Could you check a few things on this model? Use its own coordinates, in mm. Face numbers are marked on the shaded views. A direction names the side the tool comes from. Give positions to 0.01 mm unless a question says otherwise; leave off trailing zeros. Answer in a Markdown table with one row per item. Add a question column.
1. I need wall thicknesses on line 1 along Z through (x, y) = (-3.25, 29.5); line 2 along X through (y, z) = (18.5, -8.25); line 3 along X through (y, z) = (22, -2.5). Which ranges of each line are inside material? Lowest first, please. Write a range as from..to.
2. Thinking about a two-plate mould opening in Z: for the marked faces 3, 4, 5 and 6, which applies, released by +Z, released by -Z, zero draft, split by the parting line, or undercut?
3. Which directions (+Z, -Z, +X, -X, +Y, -Y) give clear straight access to the entire face, cutting with the end or side of a thin tool? Please do the marked faces 1 and 2.
4. I'm going to push flat-ended pins straight in: pin 1 Ø3.5 at (y, z) = (44.5, -1) entering from -X; pin 2 Ø0.5 at (y, z) = (30.5, -9) entering from +X; pin 3 Ø3.5 at (x, y) = (0, 21) entering from +Z. Where does each tip first touch, or does it pass through?
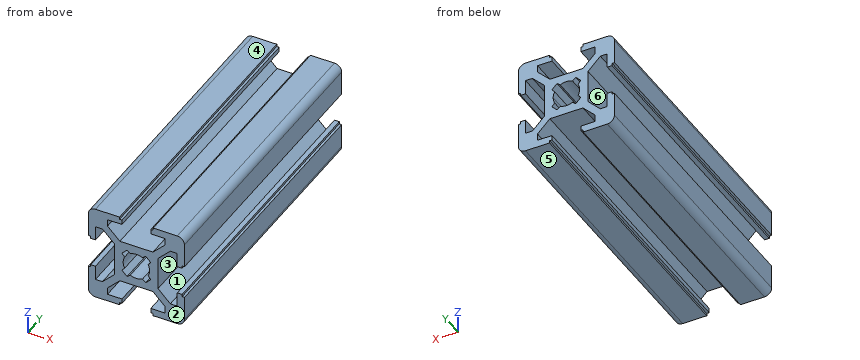
```python
from build123d import *

# Parameters (mm, degrees)
DODANIE_WYCI_GNI_CIE1_DEPTH = 60


with BuildPart() as part:
    # Szkic1 → Dodanie-wyciągnięcie1 (new body)
    with BuildSketch(Plane(origin=(0, 0, 0), x_dir=(1, 0, 0), z_dir=(0, 1, 0))):
        with BuildLine():
            Line((-7.06, 6), (-4.5, 3.440546933))
            Line((-4.5, 3.440546933), (-4.5, 4.5))
            Line((-4.5, 4.5), (-3.440546933, 4.5))
            Line((-3.440546933, 4.5), (-6, 7.06))
            Line((-6, 7.06), (-6, 8.5))
            Line((-6, 8.5), (-3, 8.5))
            Line((-3, 8.5), (-3, 9.5))
            Line((-3, 9.5), (-3.5, 9.5))
            Line((-3.5, 9.5), (-3.5, 10))
            Line((-3.5, 10), (-8.5, 10))
            ThreePointArc((-8.5, 10), (-9.560660172, 9.560660172), (-10, 8.5))
            Line((-10, 8.5), (-10, 3.5))
            Line((-10, 3.5), (-9.5, 3.5))
            Line((-9.5, 3.5), (-9.5, 3))
            Line((-9.5, 3), (-8.5, 3))
            Line((-8.5, 3), (-8.5, 6))
            Line((-8.5, 6), (-7.06, 6))
        make_face()
        with BuildLine():
            Line((4.5, 4.5), (4.5, 3.440546933))
            Line((4.5, 3.440546933), (7.06, 6))
            Line((7.06, 6), (8.5, 6))
            Line((8.5, 6), (8.5, 3))
            Line((8.5, 3), (9.5, 3))
            Line((9.5, 3), (9.5, 3.5))
            Line((9.5, 3.5), (10, 3.5))
            Line((10, 3.5), (10, 8.5))
            ThreePointArc((10, 8.5), (9.560660172, 9.560660172), (8.5, 10))
            Line((8.5, 10), (3.5, 10))
            Line((3.5, 10), (3.5, 9.5))
            Line((3.5, 9.5), (3, 9.5))
            Line((3, 9.5), (3, 8.5))
            Line((3, 8.5), (6, 8.5))
            Line((6, 8.5), (6, 7.06))
            Line((6, 7.06), (3.440546933, 4.5))
            Line((3.440546933, 4.5), (4.5, 4.5))
        make_face()
        Polygon((3.440546933, -4.5), (4.5, -4.5), (4.5, -3.440546933), (4.5, 3.440546933), (4.5, 4.5), (3.440546933, 4.5), (-3.440546933, 4.5), (-4.5, 4.5), (-4.5, 3.440546933), (-4.5, -3.440546933), (-4.5, -4.5), (-3.440546933, -4.5), align=None)
        with BuildLine():
            Line((-3.00520382, 1.944543648), (-1.944543648, 3.00520382))
            Line((-1.944543648, 3.00520382), (-1.271309214, 2.438498079))
            ThreePointArc((-1.271309214, 2.438498079), (0, 2.75), (1.271309214, 2.438498079))
            Line((1.271309214, 2.438498079), (1.944543648, 3.00520382))
            Line((1.944543648, 3.00520382), (3.00520382, 1.944543648))
            Line((3.00520382, 1.944543648), (2.438498079, 1.271309214))
            ThreePointArc((2.438498079, 1.271309214), (2.670989491, 0.654457899), (2.75, 0))
            ThreePointArc((2.75, 0), (2.670989491, -0.654457899), (2.438498079, -1.271309214))
            Line((2.438498079, -1.271309214), (3.00520382, -1.944543648))
            Line((3.00520382, -1.944543648), (1.944543648, -3.00520382))
            Line((1.944543648, -3.00520382), (1.271309214, -2.438498079))
            ThreePointArc((1.271309214, -2.438498079), (0, -2.75), (-1.271309214, -2.438498079))
            Line((-1.271309214, -2.438498079), (-1.944543648, -3.00520382))
            Line((-1.944543648, -3.00520382), (-3.00520382, -1.944543648))
            Line((-3.00520382, -1.944543648), (-2.438498079, -1.271309214))
            ThreePointArc((-2.438498079, -1.271309214), (-2.75, 0), (-2.438498079, 1.271309214))
            Line((-2.438498079, 1.271309214), (-3.00520382, 1.944543648))
        make_face(mode=Mode.SUBTRACT)
        with BuildLine():
            Line((-6, -7.06), (-3.440546933, -4.5))
            Line((-3.440546933, -4.5), (-4.5, -4.5))
            Line((-4.5, -4.5), (-4.5, -3.440546933))
            Line((-4.5, -3.440546933), (-7.06, -6))
            Line((-7.06, -6), (-8.5, -6))
            Line((-8.5, -6), (-8.5, -3))
            Line((-8.5, -3), (-9.5, -3))
            Line((-9.5, -3), (-9.5, -3.5))
            Line((-9.5, -3.5), (-10, -3.5))
            Line((-10, -3.5), (-10, -8.5))
            ThreePointArc((-10, -8.5), (-9.560660172, -9.560660172), (-8.5, -10))
            Line((-8.5, -10), (-3.5, -10))
            Line((-3.5, -10), (-3.5, -9.5))
            Line((-3.5, -9.5), (-3, -9.5))
            Line((-3, -9.5), (-3, -8.5))
            Line((-3, -8.5), (-6, -8.5))
            Line((-6, -8.5), (-6, -7.06))
        make_face()
        with BuildLine():
            Line((4.5, -3.440546933), (4.5, -4.5))
            Line((4.5, -4.5), (3.440546933, -4.5))
            Line((3.440546933, -4.5), (6, -7.06))
            Line((6, -7.06), (6, -8.5))
            Line((6, -8.5), (3, -8.5))
            Line((3, -8.5), (3, -9.5))
            Line((3, -9.5), (3.5, -9.5))
            Line((3.5, -9.5), (3.5, -10))
            Line((3.5, -10), (8.5, -10))
            ThreePointArc((8.5, -10), (9.560660172, -9.560660172), (10, -8.5))
            Line((10, -8.5), (10, -3.5))
            Line((10, -3.5), (9.5, -3.5))
            Line((9.5, -3.5), (9.5, -3))
            Line((9.5, -3), (8.5, -3))
            Line((8.5, -3), (8.5, -6))
            Line((8.5, -6), (7.06, -6))
            Line((7.06, -6), (4.5, -3.440546933))
        make_face()
    extrude(amount=DODANIE_WYCI_GNI_CIE1_DEPTH)


solid = part.part
```
Results:
| question | item | result |
|---|---|---|
| 1 | line 1 | -9.5..-8.5, -4.5..4.5, 8.5..9.5 |
| 1 | line 2 | -10..-6, 6..10 |
| 1 | line 3 | -4.5..-2.45, -1.34..-1.15, 1.15..1.34, 2.45..4.5 |
| 2 | face 3 | undercut |
| 2 | face 4 | released by +Z |
| 2 | face 5 | released by -Z |
| 2 | face 6 | undercut |
| 3 | face 1 | +Y, -Y |
| 3 | face 2 | +Z, -Z, +X, -X, -Y |
| 4 | pin 1 | x = -4.5 |
| 4 | pin 2 | x = 9.98 |
| 4 | pin 3 | z = 4.5 |
